Source: CAD feature listing. Evaluate the final solid. Frame: model axes, mm. A direction names the side the tool comes from. Round coordinates to 2 decimals unless told otherwise and drop trailing zeros. Order: outer loops, then holes, each group sorted by start corner. A loop starts at its lowest first (then second) coordinate and runs counter-clockwise, first axis right, second up. Notation, with made-up numbers: (72.5, 6.5) - (97.5, 6.5) arc R20 cw to (97.5, 23.5) - close; hole circle Ø10 at (33, -35). An arc over 180 degrees is marked (long way). Return JSON: item names as keys, results as strings. Group by question number.
1) Section A-A, the plane y = 0. Return loops of the section in (x, z).
2) Mould query, pull axis X, two halves, no side actions, for faces 1 (the cylindrical face through (76, 1, 1)), 2 (the flat face through (-78, -1, 10)), 3 (the flat face through (-75.5, -1, 10)). Classes: pulls with the +X half, pulls with the -X half, needs draft (parallel to the pull), parting line crosses it, or undercut.
3) Section C-C, the plane x = -50.5. Return loops of the section in (y, z).
4) Contact query for flat-ended pins moving along their axis: P1, Ø1.5, axis at x = 13, z = 1.5, coming from the -Y side; P2, Ø4, axis at x = -12, z = 1.5, coming from the +Y side; P3, Ø2.5, axis at y = 1, z = 1.5, coming from the +X side. Output: stop coordinate, or through.
5) Section B-B, the plane z = 9.25. Return loops of the section in (x, y), plus the area to 4 significant figures.
6) Access query for faces 4 (the flat face through (75.5, -1, 10)), 5 (the flat face through (35, 0, 2)), 6 (the cylindrical face through (-77, 1, 2)). Directions: +Z, -Z, +X, -X, +Y, -Y. A direction counts if a zero-diameter tool reaches every point of the face in a straight line with its end or side. Return the directions, or none.
7) Ray query, line 1 (Y direction, x = -37, z = 8.5); line 2 (Z direction, x = 40.5, y = 61). Return the intervals inside material, ascending. Write a range as from..to.
```python
from build123d import *

# Parameters (mm, degrees)
F0_W     = 156
F0_H     = 156
F1_DEPTH = 15
F2_W     = 151
F2_H     = 151
F3_DEPTH = 10
F4_R     = 5
F5_W     = 70
F5_H     = 5
F6_DEPTH = 5


with BuildPart() as f1:
    # F0 (on Top) → F1 (new body)
    with BuildSketch(Plane.XY):
        Rectangle(F0_W, F0_H)
    extrude(amount=F1_DEPTH)

    # F2 (on face) → F3 (cut)
    with BuildSketch(Plane.XY.offset(15)):
        Rectangle(F2_W, F2_H)
    extrude(amount=-F3_DEPTH, mode=Mode.SUBTRACT)

    # F4
    f4_edges = [f1.edges().sort_by_distance(p)[0] for p in [
        (78, 0, 0),
        (0, -78, 0),
        (-78, 0, 0),
        (0, 78, 0),
    ]]
    fillet(f4_edges, radius=F4_R)

    # F5 (on face) → F6 (cut)
    with BuildSketch(Plane(origin=(0, 0, 0), x_dir=(1, 0, 0), z_dir=(0, 0, -1))):
        Rectangle(F5_W, F5_H)
    extrude(amount=-F6_DEPTH, mode=Mode.SUBTRACT)


solid = f1.part
```
Geometry check:
{
 "1": {"outline": "(-78, 5) arc R5 ccw to (-73, 0) - (-35, 0) - (-35, 5) - (-75.5, 5) - (-75.5, 15) - (-78, 15) - close; (35, 0) - (73, 0) arc R5 ccw to (78, 5) - (78, 15) - (75.5, 15) - (75.5, 5) - (35, 5) - close"},
 "2": {"face 1": "pulls with the +X half", "face 2": "pulls with the -X half", "face 3": "undercut"},
 "3": {"outline": "(-78, 5) arc R5 ccw to (-73, 0) - (73, 0) arc R5 ccw to (78, 5) - (78, 15) - (75.5, 15) - (75.5, 5) - (-75.5, 5) - (-75.5, 15) - (-78, 15) - close"},
 "4": {"P1": "y = -77.18", "P2": "y = 77.77", "P3": "x = 77.47"},
 "5": {"outline": "(-78, -78) - (78, -78) - (78, 78) - (-78, 78) - close; hole (-75.5, -75.5) - (75.5, -75.5) - (75.5, 75.5) - (-75.5, 75.5) - close", "area": "1,535 mm2"},
 "6": {"face 4": "+Z", "face 5": "+Z, -Z", "face 6": "-Z, -X, +Y, -Y"},
 "7": {"line 1": "-78..-75.5, 75.5..78", "line 2": "0..5"}
}
